from build123d import *

# Parameters (mm, degrees)
BOSS_EXTRUDE1_DEPTH = 70
SKETCH6_R           = 1.5
CUT_EXTRUDE1_DEPTH  = 70


with BuildPart() as part:
    # Sketch1 → Boss-Extrude1 (new body)
    with BuildSketch(Plane.XY):
        Polygon((-68.951612903, 0), (-23.951612903, 0), (-23.951612903, 45), (21.048387097, 45), (21.048387097, 0), (66.048387097, 0), (66.048387097, 5), (29.048387097, 5), (29.048387097, 53), (-31.951612903, 53), (-31.951612903, 5), (-68.951612903, 5), align=None)
    extrude(amount=BOSS_EXTRUDE1_DEPTH)

    # Sketch6 → Cut-Extrude1 (cut)
    with BuildSketch(Plane(origin=(0, 5, 0), x_dir=(1, 0, 0), z_dir=(0, 1, 0))):
        with Locations(Location((-50.451612903, -14.603137979, 0), (0, 0, 180))):
            Circle(SKETCH6_R)
        with Locations(Location((-50.451612903, -54.455468389, 0), (0, 0, 180))):
            Circle(SKETCH6_R)
        with Locations(Location((47.548387097, -14.603137979, 0), (0, 0, 180))):
            Circle(SKETCH6_R)
        with Locations(Location((47.548387097, -54.455468389, 0), (0, 0, 180))):
            Circle(SKETCH6_R)
    extrude(amount=-CUT_EXTRUDE1_DEPTH, mode=Mode.SUBTRACT)


solid = part.part
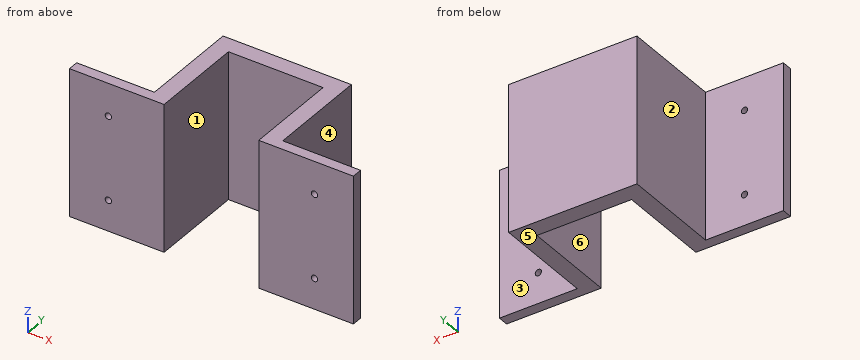
For this review, take the finished solid that the model builds, in its own axes (mm). Face numbers are marked on the shaded views. A direction names the side the tool comes from. Round coordinates to 2 decimals unless told otherwise and drop trailing zeros. Order: outer loops, then holes, each group sorted by start corner. A loop starts at its lowest first (then second) coordinate and runs counter-clockwise, first axis right, second up. Notation, with made-up numbers: M 72,63.5 L 127,63.5 A24 cw 127,100.5 Z; hole C 57,-37 d11. An arc over 180 degrees is marked long. Use a Markdown table: item, result. Add a question column.
Item 1: Mouldability with a two-part tool opening along X and no side actions: class the marked faces 4, 5 and 6 as released by +X, released by -X, zero draft, split by the parting line, or undercut.
Item 2: Add section D-D, the plane y = 48. Give the boundary of the cut face in (x, z), then the cut area to 3 significant figures.
Item 3: Insertion check: pin 1 (24 mm diameter, centred on y = 32.5, z = 19, fed in from +X); pin 2 (13.5 mm diameter, centred on x = -4.5, z = 48.5, fed in from -Y); pin 3 (22.5 mm diameter, centred on y = 21, z = 31, fed in from -X). Each pin has a flat end and moves straight along its axis. Give the tip position at first contact, or say it passes through.
Item 4: Tool access review of the marked faces 1, 2 and 3: name each direction out of +Z, -Z, +X, -X, +Y, -Y from which nothing blocks a thin tool from reaching the whole face with its end or side.
Item 5: Add section A-A, the plane y = 31.5. Give the boundary of the cut face in (x, z).
Item 6: Add section B-B, the plane z = 62. Give the boundary of the cut face in (x, y).
Item 7: Add section C-C, the plane x = -40.5. Give the boundary of the cut face in (y, z).
Item 8: To check wall thickness, follow line 1 along X through (y, z) = (6.5, 54); line 2 along Y through (x, z) = (-21, 61.5); line 3 along Y through (x, z) = (43.5, 9). State the ranges of each line that lie inside material, in increasing order.
Geometry results:
| question | item | result |
|---|---|---|
| 1 | face 4 | released by +X |
| 1 | face 5 | zero draft |
| 1 | face 6 | undercut |
| 2 | outline | M -31.95,0 L 29.05,0 L 29.05,70 L -31.95,70 Z |
| 2 | area | 4,270 mm² |
| 3 | pin 1 | stops at x = 29.05 |
| 3 | pin 2 | stops at y = 45 |
| 3 | pin 3 | stops at x = -31.95 |
| 4 | face 1 | +Z, -Z, -Y |
| 4 | face 2 | +Z, -Z, -X, +Y |
| 4 | face 3 | +Z, -Z, +X, +Y |
| 5 | outline | M -31.95,0 L -23.95,0 L -23.95,70 L -31.95,70 Z; M 21.05,0 L 29.05,0 L 29.05,70 L 21.05,70 Z |
| 6 | outline | M -68.95,0 L -23.95,0 L -23.95,45 L 21.05,45 L 21.05,0 L 66.05,0 L 66.05,5 L 29.05,5 L 29.05,53 L -31.95,53 L -31.95,5 L -68.95,5 Z |
| 7 | outline | M 0,0 L 5,0 L 5,70 L 0,70 Z |
| 8 | line 1 | x = -31.95 to -23.95, 21.05 to 29.05 |
| 8 | line 2 | y = 45 to 53 |
| 8 | line 3 | y = 0 to 5 |
